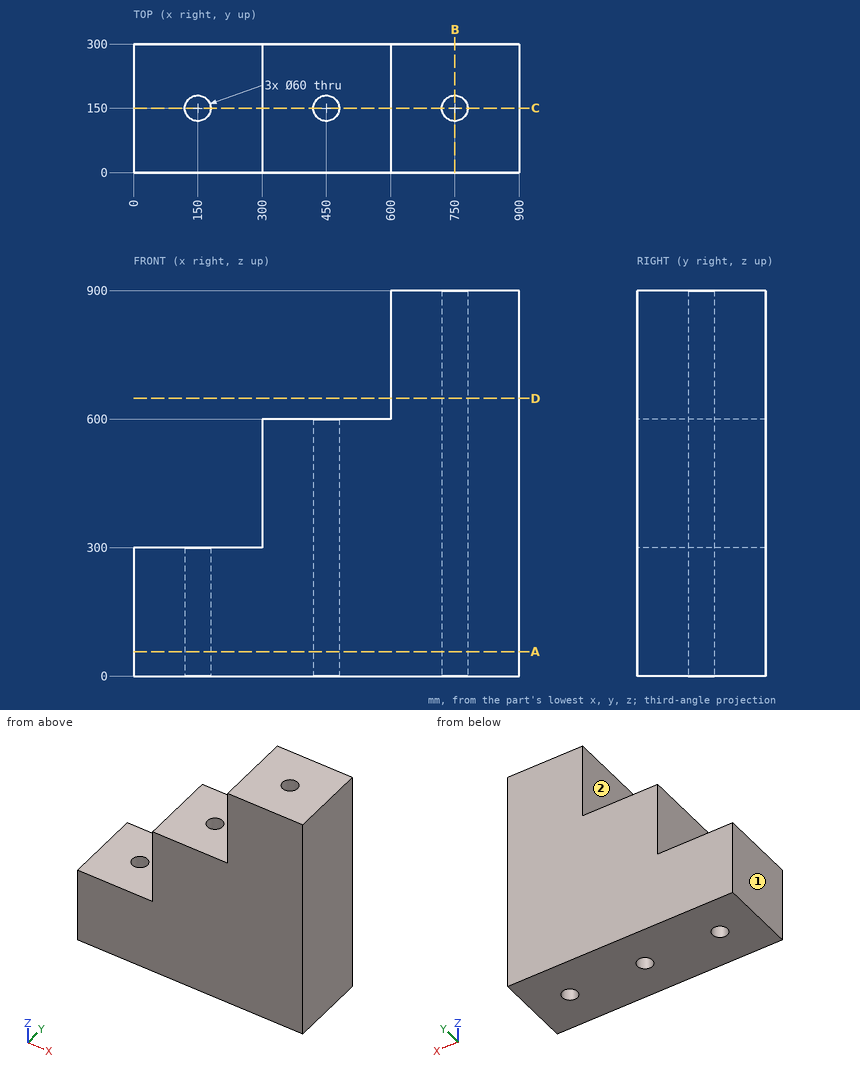
Input: dimensioned drawing with shaded views. Units: mm. Origin: part minimum x, y, z. A direction names the side the tool comes from. Give positions to 0.01 mm unless a question says otherwise; leave off trailing zeros. Write each loop counter-clockwise with the first axis right and the second up, starting at its lowest first coordinate (ties: lowest second). Pieces come first, ordered by that corner, then holes. Notation, with made-up numbers: M 36.5,77 L 43.5,77 A23 cw 43.5,88 Z; hole C 60,-18.5 d5. An arc over 180 degrees is marked long. Return JSON: item names as keys, results as strings. Group by question number.
1) Cut plane B-B, the plane x = 750. Output: boundary loops of the cut face in (y, z), plus the area to 3 significant figures.
2) Cut plane A-A, the plane z = 57. Output: boundary loops of the cut face in (x, y).
3) Cut plane D-D, the plane z = 648. Output: boundary loops of the cut face in (x, y), plus the area to 3 significant figures.
4) Material intervals for line 1 along Y through (x, z) = (450, 305); line 2 along X through (y, z) = (17, 791.5); line 3 along Z through (x, y) = (362, 266.5), sorted ascending. Write a range as [from, to].
5) Cut plane C-C, the plane y = 150. Output: boundary loops of the cut face in (x, z), plus the area to 3 significant figures.
6) Set-up query: the marked faces 1 and 2. Return all of +Z, -Z, +X, -X, +Y, -Y with unobstructed straight access to the full face (end or side cutting, diameter ignored); none if empty.
Recorded:
{
 "1": {"outline": "M 0,0 L 120,0 L 120,900 L 0,900 Z; M 180,0 L 300,0 L 300,900 L 180,900 Z", "area": "216,000 mm²"},
 "2": {"outline": "M 0,0 L 900,0 L 900,300 L 0,300 Z; hole C 150,150 d60; hole C 450,150 d60; hole C 750,150 d60"},
 "3": {"outline": "M 600,0 L 900,0 L 900,300 L 600,300 Z; hole C 750,150 d60", "area": "87,200 mm²"},
 "4": {"line 1": "y = [0, 120], [180, 300]", "line 2": "x = [600, 900]", "line 3": "z = [0, 600]"},
 "5": {"outline": "M 0,0 L 120,0 L 120,300 L 0,300 Z; M 180,0 L 420,0 L 420,600 L 300,600 L 300,300 L 180,300 Z; M 480,0 L 720,0 L 720,900 L 600,900 L 600,600 L 480,600 Z; M 780,0 L 900,0 L 900,900 L 780,900 Z", "area": "432,000 mm²"},
 "6": {"face 1": "+Z, -Z, -X, +Y, -Y", "face 2": "+Z, -X, +Y, -Y"}
}
